from build123d import *

# Parameters (mm, degrees)
BOSS_EXTRUDE1_DEPTH = 3
BOSS_EXTRUDE2_DEPTH = 4
BOSS_EXTRUDE3_DEPTH = 5


with BuildPart() as part:
    # Sketch1 → Boss-Extrude1 (new body)
    with BuildSketch(Plane.XY):
        with BuildLine():
            Line((-6.349735442, 5.345171636), (-4.997891213, 15.788269553))
            ThreePointArc((-4.997891213, 15.788269553), (0, 20.643068224), (4.997891213, 15.788269553))
            Line((4.997891213, 15.788269553), (6.349735442, 5.345171636))
            ThreePointArc((6.349735442, 5.345171636), (8.299997248, 0.006758739), (6.358432228, -5.334823296))
            Line((6.358432228, -5.334823296), (4.998253221, -16.889085995))
            ThreePointArc((4.998253221, -16.889085995), (0, -21.756931776), (-4.998253221, -16.889085995))
            Line((-4.998253221, -16.889085995), (-6.358432228, -5.334823296))
            ThreePointArc((-6.358432228, -5.334823296), (-8.299997248, 0.006758739), (-6.349735442, 5.345171636))
        make_face()
        with BuildLine():
            Line((-4.36628468, 5.088416745), (-3, 15.643068224))
            ThreePointArc((-3, 15.643068224), (0, 18.643068224), (3, 15.643068224))
            Line((3, 15.643068224), (4.36628468, 5.088416745))
            ThreePointArc((4.36628468, 5.088416745), (4.518875856, 4.540216249), (4.819678709, 4.057178471))
            ThreePointArc((4.819678709, 4.057178471), (6.299997911, 0.005130128), (4.826279884, -4.049323707))
            ThreePointArc((4.826279884, -4.049323707), (4.522307907, -4.541950371), (4.37214806, -5.100995998))
            Line((4.37214806, -5.100995998), (3, -16.756931776))
            ThreePointArc((3, -16.756931776), (0, -19.756931776), (-3, -16.756931776))
            Line((-3, -16.756931776), (-4.37214806, -5.100995998))
            ThreePointArc((-4.37214806, -5.100995998), (-4.522307907, -4.541950371), (-4.826279884, -4.049323707))
            ThreePointArc((-4.826279884, -4.049323707), (-6.299997911, 0.005130128), (-4.819678709, 4.057178471))
            ThreePointArc((-4.819678709, 4.057178471), (-4.518875856, 4.540216249), (-4.36628468, 5.088416745))
        make_face(mode=Mode.SUBTRACT)
    extrude(amount=BOSS_EXTRUDE1_DEPTH)

    # Sketch2 → Boss-Extrude2 (add)
    with BuildSketch(Plane(origin=(0, 0, 0), x_dir=(-1, 0, 0), z_dir=(0, 0, -1))):
        Polygon((10, -26.40946304), (-10, -26.40946304), (-10, 26.40946304), (-10, 71.40946304), (10, 71.40946304), (10, 26.40946304), align=None)
    extrude(amount=BOSS_EXTRUDE2_DEPTH)

    # Sketch3 → Boss-Extrude3 (add)
    with BuildSketch(Plane.XY):
        Polygon((7.25, 69.15946304), (6.1, 69.15946304), (6.1, 67.75946304), (6.1, 45.05946304), (-6.1, 45.05946304), (-6.1, 67.75946304), (-6.1, 69.15946304), (-7.25, 69.15946304), (-7.25, 43.65946304), (7.25, 43.65946304), align=None)
    extrude(amount=BOSS_EXTRUDE3_DEPTH)


solid = part.part
For this review, take the finished solid that the model builds, in its own axes (mm). A direction names the side the tool comes from. Coordinates: 2 decimals unless noted, no trailing zeros. Loops run counter-clockwise (first coordinate to the right, second up) from the corner with the lowest first, then second, coordinate; pieces in that order, holes last. Notation, with made-up numbers: (-31, 2.25) - (-23, 2.25) arc R21 cw to (-23, 38.25) - close; hole circle Ø1 at (0, -3). An arc over 180 degrees is marked (long way). Return JSON: item names as keys, results as strings.
Item 1: Insertion check: pin 1 (1.5 mm diameter, centred on x = -3, z = 3.5, fed in from +Y); pin 2 (1.5 mm diameter, centred on y = 50.5, z = 2.5, fed in from -X); pin 3 (1 mm diameter, centred on x = -1, z = 1, fed in from -Y); pin 4 (5 mm diameter, centred on y = 33, z = 3.5, fed in from +X). Each pin has a flat end and moves straight along its axis. Give the tip position at first contact, or say it passes through.
Determined:
{"pin 1": "stops at y = 45.06", "pin 2": "stops at x = -7.25", "pin 3": "stops at y = -21.73", "pin 4": "passes through"}
Item 2: Take a section at A-A (y = 51). Give the boundary of the cut face in (x, z).
Determined:
{"outline": "(-10, -4) - (10, -4) - (10, 0) - (7.25, 0) - (7.25, 5) - (6.1, 5) - (6.1, 0) - (-6.1, 0) - (-6.1, 5) - (-7.25, 5) - (-7.25, 0) - (-10, 0) - close"}
Item 3: Take a section at C-C (y = 24). Give the boundary of the cut face in (x, z), then the cut area to 3 significant figures.
Determined:
{"outline": "(-10, -4) - (10, -4) - (10, 0) - (-10, 0) - close", "area": "80.0 mm2"}
Item 4: Take a section at B-B (x = 0). Give the boundary of the cut face in (y, z), then the cut area to 3 significant figures.
Determined:
{"outline": "(-26.41, -4) - (71.41, -4) - (71.41, 0) - (45.06, 0) - (45.06, 5) - (43.66, 5) - (43.66, 0) - (20.64, 0) - (20.64, 3) - (18.64, 3) - (18.64, 0) - (-19.76, 0) - (-19.76, 3) - (-21.76, 3) - (-21.76, 0) - (-26.41, 0) - close", "area": "410 mm2"}
Item 5: Mouldability with a two-part tool opening along Y and no side actions: class faces 1 (the cylindrical face through (0.066, -19.756, 1.479)), 2 (the flat face through (7.25, 56, 2)), 3 (the flat face through (0, -26.409, -2)), 4 (the flat face through (0, 45.059, 2)) as pulls with the +Y half, pulls with the -Y half, needs draft (parallel to the pull), parting line crosses it, or undercut.
Determined:
{"face 1": "undercut", "face 2": "needs draft", "face 3": "pulls with the -Y half", "face 4": "pulls with the +Y half"}
Item 6: For faces 5 (the flat face through (6.1, 57, 2)), 6 (the flat face through (0, 23, 0)), 7 (the flat face through (-5.683, 10.494, 1.479)), 8 (the flat face through (5.664, 10.64, 1.479)), list the 3-axis set-ups (+Z, -Z, +X, -X, +Y, -Y) from which the entire face can be reached by the end or side of a thin tool; tool diameter is ignored.
Determined:
{"face 5": "+Z, +Y", "face 6": "+Z", "face 7": "+Z, -X", "face 8": "+Z, +X"}
Item 7: For line 1 (X direction, y = -17, z = 2.75); line 2 (X direction, y = 61.5, z = 3.25); line 3 (Z direction, x = -1.5, y = -20), list the stretches that pass through material, from the lowest coordinate up.
Determined:
{"line 1": "x = -4.99 to -2.99, 2.99 to 4.99", "line 2": "x = -7.25 to -6.1, 6.1 to 7.25", "line 3": "z = -4 to 3"}
